CAD build for the part. Positions are in the model's coordinates, mm. A direction names the side the tool comes from. Round coordinates to 2 decimals unless told otherwise and drop trailing zeros. Order: outer loops, then holes, each group sorted by start corner. A loop starts at its lowest first (then second) coordinate and runs counter-clockwise, first axis right, second up. Notation, with made-up numbers: M 80,7 L 116,7 A33 cw 116,46 Z; hole C 48,61 d11. An arc over 180 degrees is marked long. Answer as a JSON object with one key per item and string values. Group by question number.
```python
from build123d import *

# Parameters (mm, degrees)
CYLINDER074_R          = 1.7
CYLINDER074_DEPTH      = 50
CYLINDER074_ROLL_ANGLE = 90
CYLINDER073_R          = 1.7
CYLINDER073_DEPTH      = 50
CYLINDER073_ROLL_ANGLE = 90
BOX038_W               = 8
BOX038_H               = 21
BOX038_DEPTH           = 5
BOX037_W               = 60
BOX037_H               = 6
BOX037_DEPTH           = 5
CHAMFER005_SIZE        = 4


with BuildPart() as filament009:
    # Cylinder074 → Cylinder074 (new body)
    with BuildSketch(Plane.XY):
        Circle(CYLINDER074_R)
    extrude(amount=CYLINDER074_DEPTH)


with BuildPart() as filament009_1:
    # Cylinder074 roll: moved
    add(filament009.part.rotate(Axis((0, 0, 0), (1, 0, 0)), CYLINDER074_ROLL_ANGLE))


with BuildPart() as filament009_2:
    # Cylinder074 placement: moved
    add(filament009_1.part.moved(Location((25, 61, 67.5))))


with BuildPart() as m3_clearance002:
    # Cylinder073 → Cylinder073 (new body)
    with BuildSketch(Plane.XY):
        Circle(CYLINDER073_R)
    extrude(amount=CYLINDER073_DEPTH)


with BuildPart() as m3_clearance002_1:
    # Cylinder073 roll: moved
    add(m3_clearance002.part.rotate(Axis((0, 0, 0), (1, 0, 0)), CYLINDER073_ROLL_ANGLE))


with BuildPart() as m3_clearance002_2:
    # Cylinder073 placement: moved
    add(m3_clearance002_1.part.moved(Location((31, 61, 67.5))))

    # Fusion044: union filament009
    add(filament009_2.part)


with BuildPart() as cube035:
    # Box038 → Box038 (new body)
    with BuildSketch(Plane(origin=(81.5, 10, 65), x_dir=(1, 0, 0), z_dir=(0, 0, 1))):
        with Locations((4, 10.5)):
            Rectangle(BOX038_W, BOX038_H)
    extrude(amount=BOX038_DEPTH)


with BuildPart() as track_clamp_c:
    # Box037 → Box037 (new body)
    with BuildSketch(Plane(origin=(22, 25, 65), x_dir=(1, 0, 0), z_dir=(0, 0, 1))):
        with Locations((30, 3)):
            Rectangle(BOX037_W, BOX037_H)
    extrude(amount=BOX037_DEPTH)

    # Fusion043: union Cube035
    add(cube035.part)

    # Chamfer005
    chamfer005_edges = [track_clamp_c.edges().sort_by_distance(p)[0] for p in [
        (81.5, 25, 67.5),
    ]]
    chamfer(chamfer005_edges, length=CHAMFER005_SIZE)

    # Cut031: cut M3-clearance002
    add(m3_clearance002_2.part, mode=Mode.SUBTRACT)


solid = track_clamp_c.part
```
Item 1: Cut at B-B, the plane z = 67.5. Give the cut face in (x, y).
Item 2: Flat gauge pins, fed straight in: pin 1 Ø2.5 at (x, z) = (63.5, 66.5) entering from -Y; pin 2 Ø12 at (x, y) = (31.5, 22) entering from +Z; pin 3 Ø1.5 at (y, z) = (14.5, 67) entering from -X. Where does each tip first touch, or does it go through?
Item 3: Two-plate mould, pull along Z, no slides. Class faces 1 (the face through (62.8, 25.3, 65)), 2 (the face through (79.5, 23, 67.5)), 3 (the face through (26.57, 28.04, 66.85)): +Z half, -Z half, draft (parallel to the pull), parting line (faces both ways), or undercut.
Item 4: Cut at A-A, the plane x = 25. Give the cut face in (y, z), and give its area (3 significant figures).
Item 5: Drill centre lines: line 1 (X direction, y = 26.5, z = 67.5); line 2 (Z direction, x = 31, y = 26.95); line 3 (X direction, y = 26, z = 68.65). Where is each one in solid material? Low to high. Write a range as [from, to].
Item 6: Cut at D-D, the plane y = 23.25. Give the cut face in (x, z), and give its area (4 significant figures).
Item 7: 3-axis set-ups, long thin cutter, end or side, ignore diameter. For faces 4 (the face through (56, 25, 67)), 5 (the face through (55, 31, 67)): which of +Z, -Z, +X, -X, +Y, -Y reach the whole face in a straight line?
Item 8: Cut at C-C, the plane y = 26.75. Give the cut face in (x, z), and give its area (3 significant figures).
Response values:
{
 "1": {"outline": "M 22,25 L 23.3,25 L 23.3,31 L 22,31 Z; M 26.7,25 L 29.3,25 L 29.3,31 L 26.7,31 Z; M 32.7,25 L 77.5,25 L 81.5,21 L 81.5,10 L 89.5,10 L 89.5,31 L 32.7,31 Z"},
 "2": {"pin 1": "y = 25", "pin 2": "z = 70", "pin 3": "x = 81.5"},
 "3": {"face 1": "-Z half", "face 2": "draft", "face 3": "undercut"},
 "4": {"outline": "M 25,65 L 31,65 L 31,65.8 L 25,65.8 Z; M 25,69.2 L 31,69.2 L 31,70 L 25,70 Z", "area": "9.60 mm^2"},
 "5": {"line 1": "[22, 23.3], [26.7, 29.3], [32.7, 89.5]", "line 2": "[65, 65.8], [69.2, 70]", "line 3": "[22, 23.75], [26.25, 29.75], [32.25, 89.5]"},
 "6": {"outline": "M 79.25,65 L 89.5,65 L 89.5,70 L 79.25,70 Z", "area": "51.25 mm^2"},
 "7": {"face 4": "+Z, -Z, -X, -Y", "face 5": "+Z, -Z, +X, -X, +Y"},
 "8": {"outline": "M 22,65 L 89.5,65 L 89.5,70 L 22,70 Z; hole C 25,67.5 d3.4; hole C 31,67.5 d3.4", "area": "319 mm^2"}
}
